Build history of the part. All positions in model axes, mm. Face numbers are marked on the shaded views. A direction names the side the tool comes from. Coordinates: 2 decimals unless noted, no trailing zeros. Order: outer loops, then holes, each group sorted by start corner. A loop starts at its lowest first (then second) coordinate and runs counter-clockwise, first axis right, second up. Notation, with made-up numbers: (-33, 11.25) - (17, 11.25) arc R31 cw to (17, 41.25) - close; hole circle Ø4 at (42, 9.25). An arc over 180 degrees is marked (long way). Return JSON: item names as keys, results as strings.
from build123d import *

# Parameters (mm, degrees)
SKETCH1_R                    = 5.08
BASE_FLANGE1_DEPTH           = 1.5875
EDGE_FLANGE1_STRIP_W         = 7.8232
EDGE_FLANGE1_STRIP_H         = 1.5875
EDGE_FLANGE1_STRIP_CUT_DEPTH = 28.575
EDGE_FLANGE1_DEPTH           = 28.575


# Sheet-metal steps are written as plain solids
with BuildPart() as part:
    # Sketch1 → Base-Flange1 (new body)
    with BuildSketch(Plane.XY):
        Polygon((0, -25.4), (12.93876, -82.30362), (12.93876, -107.70362), (41.51376, -107.70362), (41.51376, -82.30362), (28.575, -25.4), (28.575, 0), (0, 0), align=None)
        with Locations((9.99998, -8.6741)):
            Circle(SKETCH1_R, mode=Mode.SUBTRACT)
    extrude(amount=-BASE_FLANGE1_DEPTH)

    # Edge-Flange1 strip (across the edge) → Edge-Flange1 strip cut (cut)
    with BuildSketch(Plane(origin=(41.51376, -107.70362, -1.5875), x_dir=(0, 1, 0), z_dir=(-1, 0, 0))):
        with Locations((-1.5875, -0.79375)):
            Rectangle(EDGE_FLANGE1_STRIP_W, EDGE_FLANGE1_STRIP_H)
    extrude(amount=EDGE_FLANGE1_STRIP_CUT_DEPTH, mode=Mode.SUBTRACT)

    # Edge-Flange1 section (across the edge) → Edge-Flange1 (add)
    with BuildSketch(Plane(origin=(41.51376, -107.70362, -1.5875), x_dir=(0, 1, 0), z_dir=(-1, 0, 0))):
        with BuildLine():
            Line((0, 0.7366), (0, 10.14222))
            Line((0, 10.14222), (1.5875, 10.14222))
            Line((1.5875, 10.14222), (1.5875, 0.7366))
            ThreePointArc((1.5875, 0.7366), (1.803245145, 0.215745145), (2.3241, 0))
            Line((2.3241, 0), (2.3241, -1.5875))
            ThreePointArc((2.3241, -1.5875), (0.68071313, -0.90678687), (0, 0.7366))
        make_face()
    extrude(amount=EDGE_FLANGE1_DEPTH)


solid = part.part
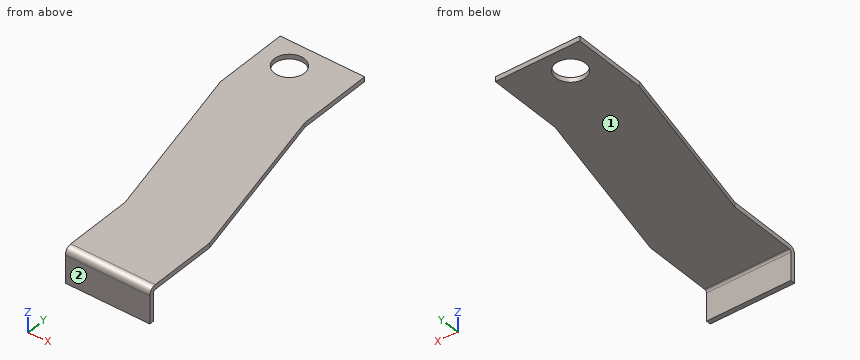
1. Tool access for the marked faces 1 and 2: list every direction of +Z, -Z, +X, -X, +Y, -Y with a clear straight run to the whole face (end or side of a thin tool).
Check values:
{"face 1": "-Z, +X, -X, +Y", "face 2": "+Z, -Z, +X, -X, -Y"}
2. Drop flat-ended pins along their axis: pin 1 (6 mm diameter, centred on x = 11.5, y = -29.5, fed in from -Z); pin 2 (4 mm diameter, centred on y = -27, z = -3, fed in from -X); pin 3 (0.5 mm diameter, centred on y = -10.5, z = -1, fed in from +X) (3 decimals); pin 4 (5 mm diameter, centred on x = 7, z = -4.5, fed in from -Y). Give the stop position or say it passes through.
Check values:
{"pin 1": "z = -1.59", "pin 2": "x = 0.04", "pin 3": "x = 28.575", "pin 4": "through"}
3. Cut at D-D on z = -5. Give the cut face in (x, y).
Check values:
{"outline": "(12.94, -107.7) - (41.51, -107.7) - (41.51, -106.12) - (12.94, -106.12) - close"}
4. Probe L1, parallel to Z at x = 24.5, y = -46.5; L2, parallel to Y at x = 33, z = -6.5; L3, parallel to X at y = -5.5, z = -0.75 (3 decimals). List the from-to ranges inside material, lowest first.
Check values:
{"L1": "-1.59 to 0", "L2": "-107.7 to -106.12", "L3": "0 to 6.034, 13.966 to 28.575"}
5. Cut at B-B on y = -10. Give the cut face in (x, z) (1 decimal), plus the area to 3 significant figures.
Check values:
{"outline": "(0, -1.6) - (5.1, -1.6) - (5.1, 0) - (0, 0) - close; (14.9, -1.6) - (28.6, -1.6) - (28.6, 0) - (14.9, 0) - close", "area": "29.8 mm²"}
6. Cut at A-A on x = 11.5. Give the cut face in (y, z).
Check values:
{"outline": "(-75.98, -1.59) - (-13.53, -1.59) - (-13.53, 0) - (-75.98, 0) - close; (-3.82, -1.59) - (0, -1.59) - (0, 0) - (-3.82, 0) - close"}
7. Cut at C-C on x = 24. Give the cut face in (y, z), plus the area to 3 significant figures.
Check values:
{"outline": "(-107.7, -11.73) - (-106.12, -11.73) - (-106.12, -2.32) arc R0.74 cw to (-105.38, -1.59) - (0, -1.59) - (0, 0) - (-105.38, 0) arc R2.32 ccw to (-107.7, -2.32) - close", "area": "186 mm²"}
